Geometry check sheet. Reference: the model listing, model coordinates, mm. A direction names the side the tool comes from. Coordinates: 2 decimals unless noted, no trailing zeros. Write each loop counter-clockwise with the first axis right and the second up, starting at its lowest first coordinate (ties: lowest second). Pieces come first, ordered by that corner, then holes. Notation, with made-up numbers: (20.5, 79) -> (68.5, 79) arc R31 ccw to (68.5, 103) -> close; hole circle Ø4 at (-7, 58). An arc over 180 degrees is marked (long way). Answer in a Markdown table with one row per item. Add a question column.
1. Scan lines: L1, parallel to Y at x = 0, z = 3.6; L2, parallel to Y at x = 0, z = 1.7; L3, parallel to Z at x = 0, y = -10. Record each from-to range of solid material in increasing order. Write a range as from..to.
2. Cross-section at D-D on y = 44.5. Record the cut outline in (x, z), and give its area (3 significant figures).
3. Set-up check for faces 1 (the cylindrical face through (-17.845, -10.079, 2.465)), 2 (the cylindrical face through (-15.22, 45.54, 2.34)): record each of +Z, -Z, +X, -X, +Y, -Y from which the full face is reachable in a straight line by a thin tool's end or side.
4. Cross-section at C-C on x = 17. Record the cut outline in (y, z).
5. Mould release check, pull along X, two halves, no side actions. Record for faces 3 (the cylindrical face through (-17.38, 26.31, 2.46)), 4 (the cylindrical face through (0, 20, 3)), 5 (the flat face through (-5, 18, 5)), 6 (the flat face through (-20, 17, 2)): pulls with the +X half, pulls with the -X half, needs draft (parallel to the pull), parting line crosses it, or undercut.
6. Cross-section at A-A on y = 18.5. Record the cut outline in (x, z).
7. Depth check by flat-ended pin: P1, Ø2.5, axis at x = 0, y = -3.5, coming from the -Z side; P2, Ø1.5, axis at x = 14, z = 2.5, coming from the +Y side; P3, Ø2, axis at x = -14, z = 2.5, coming from the +Y side; P4, Ø2, axis at x = -14, z = 2.5, coming from the -Y side. Enter the tip coordinate at first touch or a pass-through.
8. Cross-section at B-B on x = -4.5. Record the cut outline in (y, z).
Autodesk Inventor part; units mm, degrees
ref_plane "YZ Plane" through (0, 0, 0) normal (1, 0, 0) x (0, 1, 0)
ref_plane "XZ Plane" through (0, 0, 0) normal (0, 1, 0) x (-1, 0, 0)
ref_plane "XY Plane" through (0, 0, 0) normal (0, 0, 1) x (1, 0, 0)
sketch "Sketch1" plane through (0, 0, 0) normal (0, 0, 1) x (1, 0, 0)
  line L0 (20, -15) -> (-20, -15)
  line L1 (-20, -15) -> (-20, 50)
  line L2 (-20, 50) -> (20, 50)
  line L3 (20, 50) -> (20, -15)
  point P0 (0, 0)
  dimension "d0" = 40
  dimension "d1" = 65
  dimension "d27" = 15
  dimension "d28" = 20
extrude "Extrusion1" add sketch "Sketch1" along normal blind 5
sketch "Sketch5" plane through (-20, -15, 0) normal (0, -1, 0) x (1, 0, 0)
  line L0 (20, 0) -> (20, 7.6333) construction
  line L1 (0, 0) -> (0, 5) construction
  line L2 (0, 2.5) -> (40, 2.5) construction
  line L3 (40, 0) -> (40, 5) construction
  line L4 (20, 0) -> (20, 7.6333) construction
  line L5 (0, 5) -> (40, 5) construction
  point P0 (20, 2.5)
  point P1 (6, 2.5)
  point P2 (34, 2.5)
  dimension "d29" = 14
hole "Hole3" at (0, -15, 2.5) at (-14, -15, 2.5) at (14, -15, 2.5) direction (0, 1, 0) diameter 2.459 depth 8.8 tip angle 118
sketch "Sketch6" plane through (0, 0, 5) normal (0, 0, 1) x (1, 0, 0)
  line L0 (-39.4918, 7.5) -> (40.0477, 7.5) construction
  line L1 (-20, -15) -> (20, -15) construction
  line L2 (20, -15) -> (20, 50) construction
  line L3 (20, 50) -> (-20, 50) construction
  line L4 (-20, 50) -> (-20, -15) construction
  circle A0 centre (0, 7.5) radius 6.05
  line L5 (0, 63) -> (0, -28) construction
  circle A1 centre (0, 7.5) radius 11 construction
  circle A2 centre (0, -3.5) radius 1.5
  circle A3 centre (9.5263, 2) radius 1.5
  circle A4 centre (9.5263, 13) radius 1.5
  circle A5 centre (0, 18.5) radius 1.5
  circle A6 centre (-9.5263, 13) radius 1.5
  circle A7 centre (-9.5263, 2) radius 1.5
  point P0 (0, 0)
  dimension "d40" = 22
  dimension "d38" = 22.5
  dimension "d39" = 12.1
  dimension "d41" = 3
  dimension "d44" = 360
extrude "Extrusion3" cut sketch "Sketch6" against normal through all
sketch "Sketch7" plane through (0, 0, 5) normal (0, 0, 1) x (1, 0, 0)
  circle A0 centre (0, 7.5) radius 7.05
  circle A1 centre (0, 7.5) radius 6.05
  point P0 (0, 0)
  dimension "d48" = 1
extrude "Extrusion4" [suppressed]
sketch "Sketch8" plane through (-20, 50, 0) normal (0, 1, 0) x (1, 0, 0)
  circle A0 centre (6, -2.5) radius 1.2295 construction
  circle A1 centre (20, -2.5) radius 1.2295 construction
  circle A2 centre (34, -2.5) radius 1.2295 construction
  point P0 (20, 0)
hole "Hole4" at (14, 50, 2.5) at (0, 50, 2.5) at (-14, 50, 2.5) direction (0, -1, 0) diameter 2.459 depth 8.8 tip angle 118
sketch "Sketch9" plane through (0, 0, 5) normal (0, 0, 1) x (1, 0, 0)
  line L0 (17, -11) -> (-17, -11) construction
  line L1 (-17, -11) -> (-17, 27.5) construction
  line L2 (-17, 27.5) -> (17, 27.5) construction
  line L3 (17, 27.5) -> (17, -11) construction
  line L4 (17, -11) -> (-17, 27.5) construction
  line L5 (-17, -11) -> (17, 27.5) construction
  line L6 (-20, -15) -> (20, -15) construction
  line L7 (0, 63) -> (0, -28) construction
  point P0 (0, 0)
  point P1 (0, 8.25)
  dimension "d31" = 6
  dimension "d58" = 34
  dimension "d59" = 38.5
  dimension "d60" = 4
hole "Hole5" at (-17, 27.5, 5) at (17, 27.5, 5) at (17, -11, 5) at (-17, -11, 5) direction (0, 0, -1) diameter 2.5 end through all
properties part number "wheel_fix_plate_collet" material "Aluminum 6061"
Results found:
| question | item | result |
|---|---|---|
| 1 | L1 | y = -6.12..-5, -2..1.45, 13.55..17, 20..41.12 |
| 1 | L2 | y = -5.94..-5, -2..1.45, 13.55..17, 20..40.94 |
| 1 | L3 | z = 0..1.27, 3.73..5 |
| 2 | outline | (-20, 0) -> (20, 0) -> (20, 5) -> (-20, 5) -> close; hole circle Ø2.46 at (-14, 2.5); hole circle Ø2.46 at (0, 2.5); hole circle Ø2.46 at (14, 2.5) |
| 2 | area | 186 mm^2 |
| 3 | face 1 | +Z, -Z |
| 3 | face 2 | +Y |
| 4 | outline | (-15, 0) -> (-12.25, 0) -> (-12.25, 5) -> (-15, 5) -> close; (-9.75, 0) -> (26.25, 0) -> (26.25, 5) -> (-9.75, 5) -> close; (28.75, 0) -> (50, 0) -> (50, 5) -> (28.75, 5) -> close |
| 5 | face 3 | undercut |
| 5 | face 4 | undercut |
| 5 | face 5 | needs draft |
| 5 | face 6 | pulls with the -X half |
| 6 | outline | (-20, 0) -> (-1.5, 0) -> (-1.5, 5) -> (-20, 5) -> close; (1.5, 0) -> (20, 0) -> (20, 5) -> (1.5, 5) -> close |
| 7 | P1 | passes through |
| 7 | P2 | stops at y = 40.91 |
| 7 | P3 | stops at y = 41.06 |
| 7 | P4 | stops at y = -6.06 |
| 8 | outline | (-15, 0) -> (3.46, 0) -> (3.46, 5) -> (-15, 5) -> close; (11.54, 0) -> (50, 0) -> (50, 5) -> (11.54, 5) -> close |
